from build123d import *

# Parameters (mm, degrees)
F0_W      = 63
F0_H      = 54
F1_DEPTH  = 4
F2_W      = 63
F2_H      = 54
F3_DEPTH  = 8
F6_R      = 2
F7_DEPTH  = 3
F8_D      = 2.5
F8_DEPTH  = 4.5
F8_TIP    = 0.7510757738
F10_D     = 2.5
F10_DEPTH = 4.5
F10_TIP   = 0.7510757738
F12_D     = 5
F12_DEPTH = 3
F12_TIP   = 1.5021515476
F14_D     = 5
F14_DEPTH = 3
F14_TIP   = 1.5021515476
F15_D     = 2.5
F15_DEPTH = 4.5
F15_TIP   = 0.7510757738
F17_D     = 5
F17_DEPTH = 3
F17_TIP   = 1.5021515476
F18_R     = 1.5
F19_DEPTH = 12


with BuildPart() as f1:
    # F0 (on Top) → F1 (new body)
    with BuildSketch(Plane.XY):
        with Locations((31.5, 27)):
            Rectangle(F0_W, F0_H)
    extrude(amount=F1_DEPTH)

    # F2 (on face) → F3 (join)
    with BuildSketch(Plane.XY.offset(4)):
        with Locations((31.5, 27)):
            Rectangle(F2_W, F2_H)
        Polygon((3, 48), (6, 51), (57, 51), (60, 48), (60, 6), (57, 3), (6, 3), (3, 6), align=None, mode=Mode.SUBTRACT)
    extrude(amount=F3_DEPTH)

    # F6 (on face) → F7 (cut)
    with BuildSketch(Plane(origin=(0, 54, 0), x_dir=(-1, 0, 0), z_dir=(0, 1, 0))):
        with Locations((-43, 6)):
            Circle(F6_R)
        with Locations((-51, 6)):
            Circle(F6_R)
    extrude(amount=-F7_DEPTH, mode=Mode.SUBTRACT)

    # F8
    with Locations(Plane.XZ):
        with Locations((26, 6), (37, 6)):
            Hole(F8_D / 2, depth=F8_DEPTH)
            with Locations((0, 0, -(F8_DEPTH + F8_TIP / 2))):  # 118° drill point
                Cone(0, F8_D / 2, F8_TIP, mode=Mode.SUBTRACT)

    # F10
    with Locations(Plane(origin=(0, 0, 0), x_dir=(0, -1, 0), z_dir=(-1, 0, 0))):
        with Locations((-32.5, 6), (-21.5, 6)):
            Hole(F10_D / 2, depth=F10_DEPTH)
            with Locations((0, 0, -(F10_DEPTH + F10_TIP / 2))):  # 118° drill point
                Cone(0, F10_D / 2, F10_TIP, mode=Mode.SUBTRACT)

    # F12
    with Locations(Plane(origin=(0, 0, 0), x_dir=(0, -1, 0), z_dir=(-1, 0, 0))):
        with Locations((-27, 6)):
            Hole(F12_D / 2, depth=F12_DEPTH)
            with Locations((0, 0, -(F12_DEPTH + F12_TIP / 2))):  # 118° drill point
                Cone(0, F12_D / 2, F12_TIP, mode=Mode.SUBTRACT)

    # F14
    with Locations(Plane.XZ):
        with Locations((31.5, 6)):
            Hole(F14_D / 2, depth=F14_DEPTH)
            with Locations((0, 0, -(F14_DEPTH + F14_TIP / 2))):  # 118° drill point
                Cone(0, F14_D / 2, F14_TIP, mode=Mode.SUBTRACT)

    # F15
    with Locations(Plane.YZ.offset(63)):
        with Locations((21.5, 6), (32.5, 6)):
            Hole(F15_D / 2, depth=F15_DEPTH)
            with Locations((0, 0, -(F15_DEPTH + F15_TIP / 2))):  # 118° drill point
                Cone(0, F15_D / 2, F15_TIP, mode=Mode.SUBTRACT)

    # F17
    with Locations(Plane.YZ.offset(63)):
        with Locations((27, 6)):
            Hole(F17_D / 2, depth=F17_DEPTH)
            with Locations((0, 0, -(F17_DEPTH + F17_TIP / 2))):  # 118° drill point
                Cone(0, F17_D / 2, F17_TIP, mode=Mode.SUBTRACT)

    # F18 (on face) → F19 (cut)
    with BuildSketch(Plane.XY.offset(12)):
        with Locations((2.5, 51.5)):
            Circle(F18_R)
        with Locations((60.5, 51.5)):
            Circle(F18_R)
        with Locations((2.5, 2.5)):
            Circle(F18_R)
        with Locations((60.5, 2.5)):
            Circle(F18_R)
    extrude(amount=-F19_DEPTH, mode=Mode.SUBTRACT)


solid = f1.part
Model file for the job. Use its own axes, mm. A direction names the side the tool comes from. Give positions to 0.01 mm unless a question says otherwise; leave off trailing zeros. Order: outer loops, then holes, each group sorted by start corner. A loop starts at its lowest first (then second) coordinate and runs counter-clockwise, first axis right, second up. Notation, with made-up numbers: (-17, 61) - (4, 61) arc R19 ccw to (4, 84) - close; hole circle Ø10 at (59, 33). An arc over 180 degrees is marked (long way). Return JSON: item names as keys, results as strings.
1) Flat gauge pins, fed straight in: P1, Ø4, axis at x = 30.5, z = 9, coming from the -Y side; P2, Ø3, axis at x = 31.5, z = 6, coming from the -Y side; P3, Ø4.5, axis at y = 27, z = 6, coming from the +X side; P4, Ø2, axis at x = 39.5, y = 39.5, coming from the +Z side. Where does each tip first touch, or does it go through?
Geometry says:
{"P1": "y = 0", "P2": "y = 51", "P3": "x = 59.85", "P4": "z = 4"}
2) Cut at C-C, the plane z = 11.25. Give the cut face in (x, y).
Geometry says:
{"outline": "(0, 0) - (63, 0) - (63, 54) - (0, 54) - close; hole circle Ø3 at (2.5, 2.5); hole circle Ø3 at (2.5, 51.5); hole (3, 6) - (6, 3) - (57, 3) - (60, 6) - (60, 48) - (57, 51) - (6, 51) - (3, 48) - close; hole circle Ø3 at (60.5, 2.5); hole circle Ø3 at (60.5, 51.5)"}
3) Cut at D-D, the plane y = 49. Give the cut face in (x, z).
Geometry says:
{"outline": "(0, 0) - (63, 0) - (63, 12) - (59, 12) - (59, 4) - (4, 4) - (4, 12) - (0, 12) - close"}
4) 3-axis set-ups, long thin cutter, end or side, ignore diameter. For faces 1 (the flat face through (58, 50, 8)), 2 (the cylindrical face through (61.48, 28.84, 7.69)), 3 (the cylindrical face through (2.175, 1.036, 6.084)), 4 (the cylindrical face through (1.52, 25.16, 7.69)): which of +Z, -Z, +X, -X, +Y, -Y reach the whole face in a straight line?
Geometry says:
{"face 1": "+Z", "face 2": "+X", "face 3": "+Z, -Z", "face 4": "-X"}
5) Probe line 1 (X direction, y = 53.15, z = 6); line 2 (X direction, y = 12, z = 5.75); line 3 (Z direction, x = 43, y = 52). List the from-to ranges inside material, lowest first. Write a range as from..to.
Geometry says:
{"line 1": "0..41, 45..49, 53..63", "line 2": "0..3, 60..63", "line 3": "0..4, 8..12"}
6) Cut at B-B, the plane y = 21.5. Give the cut face in (x, z), plus the area to 3 significant figures.
Geometry says:
{"outline": "(0, 0) - (63, 0) - (63, 4.75) - (60, 4.75) - (60, 4) - (3, 4) - (3, 4.75) - (0, 4.75) - close; (0, 7.25) - (3, 7.25) - (3, 12) - (0, 12) - close; (60, 7.25) - (63, 7.25) - (63, 12) - (60, 12) - close", "area": "285 mm²"}
7) Pull direction Y, two halves, no side cores. Call faces 5 (the flat face through (31, 54, 6)), 6 (the cylindrical face through (34, 2, 6)), 7 (the flat face through (60, 27, 9)): pulls with the +Y half, pulls with the -Y half, needs draft (parallel to the pull), parting line crosses it, or undercut.
Geometry says:
{"face 5": "pulls with the +Y half", "face 6": "needs draft", "face 7": "undercut"}
8) Cut at A-A, the plane x = 26. Give the cut face in (y, z).
Geometry says:
{"outline": "(0, 0) - (54, 0) - (54, 12) - (51, 12) - (51, 4) - (3, 4) - (3, 4.75) - (0, 4.75) - close; (0, 7.25) - (3, 7.25) - (3, 12) - (0, 12) - close"}
